Geometry: final body of the model. Coordinates: model frame, mm. A direction names the side the tool comes from. Give positions to 0.01 mm unless a question says otherwise; leave off trailing zeros. Write each loop counter-clockwise with the first axis right and the second up, starting at its lowest first coordinate (ties: lowest second). Pieces come first, ordered by that corner, then holes.
Q1. Line query: line 1 (Y direction, x = 79, z = 2.3); line 2 (Y direction, x = 20, z = 2); line 3 (Y direction, x = 150, z = 7). Output: solid intervals per line, ascending.
Q2. Mould query, pull axis X, two halves, no side actions, for faces 1 (the flat face through (0, 89, 27)), 2 (the flat face through (64, 177, 29)), 3 (the flat face through (64, 180, 27)), 4 (the flat face through (160, 29, 33)). Classes: +X half, -X half, draft (parallel to the pull), parting line (faces both ways), or undercut.
Q3. Pin query (flat end, axial travel): pin 1 Ø9 at (x, y) = (105, 20) entering from +Z; pin 2 Ø3.5 at (y, z) = (179, 41.5) entering from +X; pin 3 Ø1.5 at (x, y) = (25, 178.5) entering from +Z; pin 4 Ø4.5 at (x, y) = (35, 85) entering from -Z. Return the tip coordinate at first contact, or that it passes through.
Q4. Section A-A (y = 85). Return the cut outline in (x, z), plus the area to 4 significant figures.
Q5. Reachability of faces 5 (the flat face through (3, 89, 29)), 6 (the cylindrical face through (102.253, 20.121, 1.479)), 7 (the flat face through (145, 75, 27)) from +Z, -Z, +X, -X, +Y, -Y: full face, straight path, thin tool, end or side. Return the list, or none.
Q6. Section D-D (x = 20). Return the cut outline in (y, z), plus the area to 4 significant figures.
Q7. Section C-C (z = 42.5). Return the cut outline in (x, y).
Q8. Section B-B (x = 144). Return the cut outline in (y, z), plus the area to 3 significant figures.
from build123d import *

# Parameters (mm, degrees)
BOX021_W          = 150
BOX021_H          = 37
BOX021_DEPTH      = 45
BOX018_W          = 15
BOX018_H          = 20
BOX018_DEPTH      = 20
BOX017_W          = 17
BOX017_H          = 20
BOX017_DEPTH      = 28
CYLINDER015_R     = 2.75
CYLINDER015_DEPTH = 10
CYLINDER016_R     = 2.75
CYLINDER016_DEPTH = 10
CYLINDER017_R     = 2.75
CYLINDER017_DEPTH = 10
CYLINDER018_R     = 5.5
CYLINDER018_DEPTH = 10
CYLINDER014_R     = 2.75
CYLINDER014_DEPTH = 10
BOX016_W          = 30
BOX016_H          = 69
BOX016_DEPTH      = 55
BOX015_W          = 124
BOX015_H          = 174
BOX015_DEPTH      = 55
BOX014_W          = 30
BOX014_H          = 105
BOX014_DEPTH      = 55
BOX009_W          = 160
BOX009_H          = 180
BOX009_DEPTH      = 55


with BuildPart() as obj1:
    # Box021 → Box021 (new body)
    with BuildSketch(Plane(origin=(10, 30, 0), x_dir=(1, 0, 0), z_dir=(0, 0, 1))):
        with Locations((75, 18.5)):
            Rectangle(BOX021_W, BOX021_H)
    extrude(amount=BOX021_DEPTH)


with BuildPart() as obj2:
    # Box018 → Box018 (new body)
    with BuildSketch(Plane(origin=(17, 170, 35), x_dir=(1, 0, 0), z_dir=(0, 0, 1))):
        with Locations((7.5, 10)):
            Rectangle(BOX018_W, BOX018_H)
    extrude(amount=BOX018_DEPTH)


with BuildPart() as fusion012:
    # Box017 → Box017 (new body)
    with BuildSketch(Plane(origin=(97, 170, 27), x_dir=(1, 0, 0), z_dir=(0, 0, 1))):
        with Locations((8.5, 10)):
            Rectangle(BOX017_W, BOX017_H)
    extrude(amount=BOX017_DEPTH)

    # Fusion012: union obj2
    add(obj2.part)


with BuildPart() as zylinder001:
    # Cylinder015 → Cylinder015 (new body)
    with BuildSketch(Plane(origin=(105, 20, -3), x_dir=(1, 0, 0), z_dir=(0, 0, 1))):
        Circle(CYLINDER015_R)
    extrude(amount=CYLINDER015_DEPTH)


with BuildPart() as zylinder002:
    # Cylinder016 → Cylinder016 (new body)
    with BuildSketch(Plane(origin=(79, 159, -3), x_dir=(1, 0, 0), z_dir=(0, 0, 1))):
        Circle(CYLINDER016_R)
    extrude(amount=CYLINDER016_DEPTH)


with BuildPart() as zylinder003:
    # Cylinder017 → Cylinder017 (new body)
    with BuildSketch(Plane(origin=(35, 85, -3), x_dir=(1, 0, 0), z_dir=(0, 0, 1))):
        Circle(CYLINDER017_R)
    extrude(amount=CYLINDER017_DEPTH)


with BuildPart() as zylinder004:
    # Cylinder018 → Cylinder018 (new body)
    with BuildSketch(Plane(origin=(60, 150, -3), x_dir=(1, 0, 0), z_dir=(0, 0, 1))):
        Circle(CYLINDER018_R)
    extrude(amount=CYLINDER018_DEPTH)


with BuildPart() as fusion008:
    # Cylinder014 → Cylinder014 (new body)
    with BuildSketch(Plane(origin=(20, 20, -3), x_dir=(1, 0, 0), z_dir=(0, 0, 1))):
        Circle(CYLINDER014_R)
    extrude(amount=CYLINDER014_DEPTH)

    # Fusion008: union Zylinder001, Zylinder002, Zylinder003, Zylinder004
    add(zylinder001.part)
    add(zylinder002.part)
    add(zylinder003.part)
    add(zylinder004.part)


with BuildPart() as obj3:
    # Box016 → Box016 (new body)
    with BuildSketch(Plane(origin=(127, 3, 3), x_dir=(1, 0, 0), z_dir=(0, 0, 1))):
        with Locations((15, 34.5)):
            Rectangle(BOX016_W, BOX016_H)
    extrude(amount=BOX016_DEPTH)


with BuildPart() as fusion011:
    # Box015 → Box015 (new body)
    with BuildSketch(Plane(origin=(3, 3, 3), x_dir=(1, 0, 0), z_dir=(0, 0, 1))):
        with Locations((62, 87)):
            Rectangle(BOX015_W, BOX015_H)
    extrude(amount=BOX015_DEPTH)

    # Fusion011: union obj3
    add(obj3.part)


with BuildPart() as obj4:
    # Box014 → Box014 (new body)
    with BuildSketch(Plane(origin=(130, 75, 0), x_dir=(1, 0, 0), z_dir=(0, 0, 1))):
        with Locations((15, 52.5)):
            Rectangle(BOX014_W, BOX014_H)
    extrude(amount=BOX014_DEPTH)


with BuildPart() as cut017:
    # Box009 → Box009 (new body)
    with BuildSketch(Plane.XY):
        with Locations((80, 90)):
            Rectangle(BOX009_W, BOX009_H)
    extrude(amount=BOX009_DEPTH)

    # Cut012: cut obj4
    add(obj4.part, mode=Mode.SUBTRACT)

    # Cut013: cut Fusion011
    add(fusion011.part, mode=Mode.SUBTRACT)

    # Cut014: cut Fusion008
    add(fusion008.part, mode=Mode.SUBTRACT)

    # Cut015: cut Fusion012
    add(fusion012.part, mode=Mode.SUBTRACT)

    # Cut017: cut obj1
    add(obj1.part, mode=Mode.SUBTRACT)


solid = cut017.part
Computed:
1. line 1: y = 0 to 30, 67 to 156.25, 161.75 to 180
1. line 2: y = 0 to 17.25, 22.75 to 30, 67 to 180
1. line 3: y = 0 to 3, 72 to 75
2. face 1: -X half
2. face 2: undercut
2. face 3: draft
2. face 4: +X half
3. pin 1: stops at z = 3
3. pin 2: stops at x = 130
3. pin 3: stops at z = 35
3. pin 4: passes through
4. outline: (0, 0) - (32.25, 0) - (32.25, 3) - (3, 3) - (3, 55) - (0, 55) - close; (37.75, 0) - (130, 0) - (130, 55) - (127, 55) - (127, 3) - (37.75, 3) - close
4. area: 685.5 mm2
5. face 5: +Z
5. face 6: +Z, -Z
5. face 7: +Z, -Z, +X, +Y
6. outline: (0, 0) - (17.25, 0) - (17.25, 3) - (3, 3) - (3, 55) - (0, 55) - close; (22.75, 0) - (30, 0) - (30, 3) - (22.75, 3) - close; (67, 0) - (180, 0) - (180, 35) - (177, 35) - (177, 3) - (67, 3) - close
6. area: 664.5 mm2
7. outline: (0, 0) - (160, 0) - (160, 30) - (157, 30) - (157, 3) - (3, 3) - (3, 177) - (17, 177) - (17, 180) - (0, 180) - close; (32, 177) - (97, 177) - (97, 180) - (32, 180) - close; (114, 177) - (127, 177) - (127, 72) - (157, 72) - (157, 67) - (160, 67) - (160, 75) - (130, 75) - (130, 180) - (114, 180) - close
8. outline: (0, 0) - (30, 0) - (30, 3) - (3, 3) - (3, 55) - (0, 55) - close; (67, 0) - (75, 0) - (75, 55) - (72, 55) - (72, 3) - (67, 3) - close
8. area: 426 mm2
